Check sheet for the drawn part. Datum: minimum x, y, z corner. Units: mm. Give positions to 0.01 mm unless a question says otherwise; leave off trailing zeros. Loops run counter-clockwise (first coordinate to the right, second up) from the corner with the lowest first, then second, coordinate; pieces in that order, holes last. Notation, with made-up numbers: (40, 83.5) - (70, 83.5) arc R20 cw to (70, 90.5) - close; hole circle Ø9 at (86.25, 72.5). An arc over 180 degrees is marked (long way). Use one line per item in the form item = value.
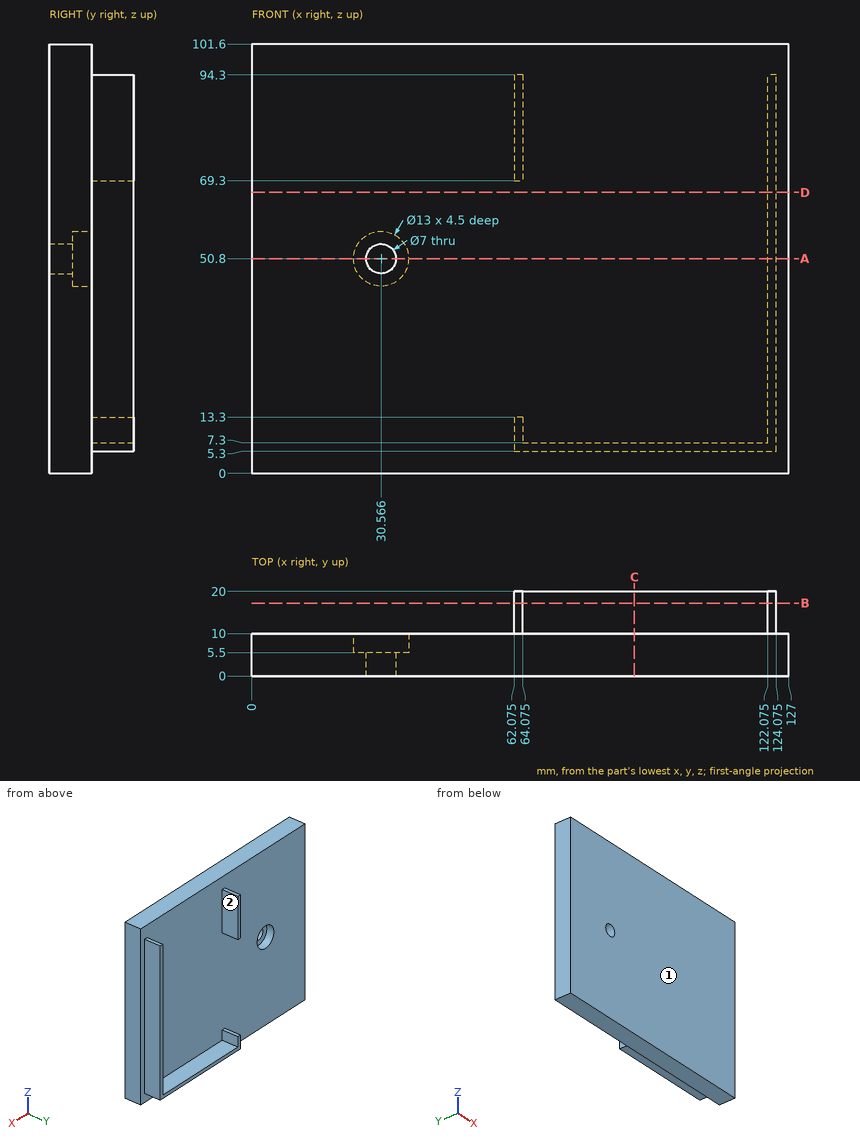
Item 1: Mould release check, pull along X, two halves, no side actions. Record for the marked faces 1 and 2: released by +X, released by -X, zero draft, split by the parting line, or undercut.
Answer block:
face_1 = zero draft
face_2 = undercut
Item 2: Section check C-C on x = 90.5. Record the boundary of the cut face in (y, z).
Answer block:
outline = (0, 0) - (10, 0) - (10, 5.3) - (20, 5.3) - (20, 7.3) - (10, 7.3) - (10, 101.6) - (0, 101.6) - close
Item 3: Gauge pin test, flat ends, axial feed: P1, Ø1.6, axis at x = 63, y = 15.5, coming from the +Z side; P2, Ø0.6, axis at x = 63, y = 14.5, coming from the -Z side; P3, Ø3, axis at y = 15, z = 80.5, coming from the -X side (1 decimal); P4, Ø1, axis at x = 50.5, y = 6, coming from the -Z side. Record the tip position at first contact, or that the pin passes through.
Answer block:
P1 = 94.3
P2 = 5.3
P3 = 62.1
P4 = 0
Item 4: Section check D-D on z = 66.5. Record the boundary of the cut face in (x, y) (1 decimal).
Answer block:
outline = (0, 0) - (127, 0) - (127, 10) - (124.1, 10) - (124.1, 20) - (122.1, 20) - (122.1, 10) - (0, 10) - close
Item 5: Section check A-A on z = 50.8. Record the boundary of the cut face in (x, y) (1 decimal).
Answer block:
outline = (0, 0) - (27.1, 0) - (27.1, 5.5) - (24.1, 5.5) - (24.1, 10) - (0, 10) - close; (34.1, 0) - (127, 0) - (127, 10) - (124.1, 10) - (124.1, 20) - (122.1, 20) - (122.1, 10) - (37.1, 10) - (37.1, 5.5) - (34.1, 5.5) - close
Item 6: Thickness scan on L1, parallel to X at y = 4.35, z = 50.8 (1 decimal); L2, parallel to X at y = 7.6, z = 50.8 (1 decimal); L3, parallel to Y at x = 57, z = 90.5. Record the ranges inside material, lowest first.
Answer block:
L1 = 0 to 27.1, 34.1 to 127
L2 = 0 to 24.1, 37.1 to 127
L3 = 0 to 10
Item 7: Section check B-B on y = 17.25. Record the boundary of the cut face in (x, z) (1 decimal), then the cut area to 3 significant figures.
Answer block:
outline = (62.1, 5.3) - (124.1, 5.3) - (124.1, 94.3) - (122.1, 94.3) - (122.1, 7.3) - (64.1, 7.3) - (64.1, 13.3) - (62.1, 13.3) - close; (62.1, 69.3) - (64.1, 69.3) - (64.1, 94.3) - (62.1, 94.3) - close
area = 360 mm2
